from build123d import *

# Parameters (mm, degrees)
SKETCH_1_R          = 9.5
EXTRUDE_1_DEPTH     = 6
SKETCH_2_R          = 8.5
CUT_EXTRUDE_1_DEPTH = 1
CUT_EXTRUDE_START   = -1
SKETCH_3_R          = 8.5
CUT_EXTRUDE_2_DEPTH = 1
SKETCH_4_R          = 5
EXTRUDE_4_DEPTH     = 1
EXTRUDE_START       = 1
SKETCH_6_R          = 5
EXTRUDE_5_DEPTH     = 1
SKETCH_7_R          = 3
CUT_EXTRUDE_3_DEPTH = 6


with BuildPart() as part:
    # 스케치1 → 돌출1 (new body)
    with BuildSketch(Plane.XY):
        Circle(SKETCH_1_R)
    extrude(amount=EXTRUDE_1_DEPTH)

    # 스케치2 → 컷-돌출1 (cut)
    with BuildSketch(Plane.XY.offset(6)):
        Circle(SKETCH_2_R)
    extrude(amount=-CUT_EXTRUDE_1_DEPTH, mode=Mode.SUBTRACT)

    # 스케치3 → 컷-돌출2 (cut)
    with BuildSketch(Plane(origin=(0, 0, 0), x_dir=(-1, 0, 0), z_dir=(0, 0, -1)).offset(CUT_EXTRUDE_START)):
        with Locations(Location((0, 0, 0), (0, 0, 180))):
            Circle(SKETCH_3_R)
    extrude(amount=CUT_EXTRUDE_2_DEPTH, mode=Mode.SUBTRACT)

    # 스케치4 → 돌출4 (add)
    with BuildSketch(Plane.XY.offset(5)):
        Circle(SKETCH_4_R)
    extrude(amount=EXTRUDE_4_DEPTH)

    # 스케치6 → 돌출5 (add)
    with BuildSketch(Plane(origin=(0, 0, 1), x_dir=(-1, 0, 0), z_dir=(0, 0, -1)).offset(EXTRUDE_START)):
        with Locations(Location((0, 0, 0), (0, 0, 180))):
            Circle(SKETCH_6_R)
    extrude(amount=-EXTRUDE_5_DEPTH)

    # 스케치7 → 컷-돌출3 (cut)
    with BuildSketch(Plane.XY.offset(6)):
        Circle(SKETCH_7_R)
    extrude(amount=-CUT_EXTRUDE_3_DEPTH, mode=Mode.SUBTRACT)


solid = part.part
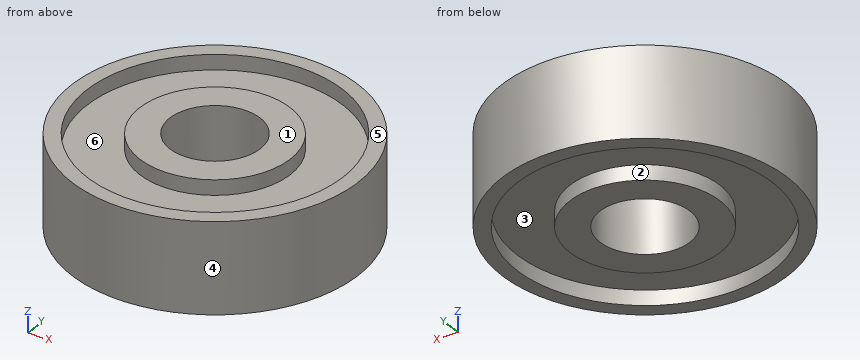
Verification items for the finished model (mm, model axes). Face numbers are marked on the shaded views. A direction names the side the tool comes from. Give positions to 0.01 mm unless a question says otherwise; leave off trailing zeros. Write each loop counter-clockwise with the first axis right and the second up, starting at its lowest first coordinate (ties: lowest second). Pieces come first, ordered by that corner, then holes. Notation, with made-up numbers: M 63,37 L 90,37 A21 cw 90,72 Z; hole C 2,-29.5 d9. An arc over 180 degrees is marked long. Use CSV: the item, a comma, the result in double quotes.
1) Cross-section at B-B (z = 5.25). Enter the section's corners in (x, y).
Final values:
outline,"C 0,0 d19; C 0,0 d10; hole C 0,0 d17; hole C 0,0 d6"
2) Cross-section at D-D (y = 4.75). Enter the section's corners in (x, z), plus the area to 3 significant figures.
Final values:
outline,"M -8.23,0 L -7.05,0 L -7.05,1 L -1.56,1 L -1.56,0 L 1.56,0 L 1.56,1 L 7.05,1 L 7.05,0 L 8.23,0 L 8.23,6 L 7.05,6 L 7.05,5 L 1.56,5 L 1.56,6 L -1.56,6 L -1.56,5 L -7.05,5 L -7.05,6 L -8.23,6 Z"
area,"76.8 mm²"
3) Cross-section at A-A (x = 0). Enter the section's corners in (y, z), plus the area to 3 significant figures.
Final values:
outline,"M -9.5,0 L -8.5,0 L -8.5,1 L -5,1 L -5,0 L -3,0 L -3,6 L -5,6 L -5,5 L -8.5,5 L -8.5,6 L -9.5,6 Z; M 3,0 L 5,0 L 5,1 L 8.5,1 L 8.5,0 L 9.5,0 L 9.5,6 L 8.5,6 L 8.5,5 L 5,5 L 5,6 L 3,6 Z"
area,"64.0 mm²"
4) Release check for a two-part mould opening along Y. For the marked faces 1, 2, 3 and 4 record: released by +Y, released by -Y, zero draft, split by the parting line, or undercut.
Final values:
face 1,"zero draft"
face 2,"undercut"
face 3,"undercut"
face 4,"split by the parting line"
5) Material ranges on line 1 along Y through (x, z) = (0, 5.7); line 2 along Y through (x, z) = (0, 3.1); line 3 along X through (y, z) = (4.25, 5.35), recorded low to high.
Final values:
line 1,"-9.5 to -8.5, -5 to -3, 3 to 5, 8.5 to 9.5"
line 2,"-9.5 to -3, 3 to 9.5"
line 3,"-8.5 to -7.36, -2.63 to 2.63, 7.36 to 8.5"
6) Access from +Z, -Z, +X, -X, +Y, -Y to the whole of each face (thin tool, end or side, straight path). Record for the marked faces 5 and 6.
Final values:
face 5,"+Z, +X, -X, +Y, -Y"
face 6,"+Z"
7) Go/stop test with flat-tipped pins: pin 1 Ø1 at (y, z) = (1.5, 3) entering from +X; pin 2 Ø1.5 at (x, z) = (6.5, 5) entering from +Y; pin 3 Ø5.5 at (x, y) = (0, 0) entering from -Z. Record where each tip stops, or that it passes through.
Final values:
pin 1,"x = 9.45"
pin 2,"y = 7.56"
pin 3,"through"
